Read the model definition and answer for the solid it produces. Units are mm, in the model's axes. Face numbers are marked on the shaded views. A direction names the side the tool comes from. Coordinates: 2 decimals unless noted, no trailing zeros. Loops run counter-clockwise (first coordinate to the right, second up) from the corner with the lowest first, then second, coordinate; pieces in that order, holes last. Notation, with made-up numbers: (30, -3.75) -> (54, -3.75) arc R21 ccw to (54, 34.25) -> close; hole circle Ø7 at (25.25, 83.25). An arc over 180 degrees is marked (long way). Answer in a Markdown table with one row per item.
```python
from build123d import *

# Parameters (mm, degrees)
ESQUISSE1_R          = 2
ESQUISSE1_R_2        = 1.5
BOSS_EXTRU_1_DEPTH   = 39.58852
BOSS_EXTRU_1_2_DEPTH = 39.58852
BOSS_EXTRU_2_DEPTH   = 20


with BuildPart() as part:
    # Esquisse1 → Boss.-Extru.1 (new body)
    with BuildSketch(Plane.XY):
        with Locations(Location((0, 3.882050808, 0), (0, 0, 180))):
            Circle(ESQUISSE1_R)
        with Locations(Location((0, 3.882050808, 0), (0, 0, 180))):
            Circle(ESQUISSE1_R_2, mode=Mode.SUBTRACT)
    extrude(amount=BOSS_EXTRU_1_DEPTH)



with BuildPart() as body_2:
    # Esquisse1 → Boss.-Extru.1 2 (new body)
    with BuildSketch(Plane.XY):
        with Locations(Location((0, -3.882050808, 0), (0, 0, 180))):
            Circle(ESQUISSE1_R)
        with Locations((0, -3.882050808)):
            Circle(ESQUISSE1_R_2, mode=Mode.SUBTRACT)
    extrude(amount=BOSS_EXTRU_1_2_DEPTH)


with BuildPart() as part_1:
    add(part.part)

    add(body_2.part)  # Boss.-Extru.2 merges body 2
    # Esquisse1<3> → Boss.-Extru.2 (add)
    with BuildSketch(Plane.XY):
        with BuildLine():
            ThreePointArc((-1, -2.15), (0, -1.882050808), (1, -2.15))
            Line((1, -2.15), (1, 2.15))
            ThreePointArc((1, 2.15), (0, 1.882050808), (-1, 2.15))
            Line((-1, 2.15), (-1, -2.15))
        make_face()
    extrude(amount=BOSS_EXTRU_2_DEPTH)


solid = part_1.part
```
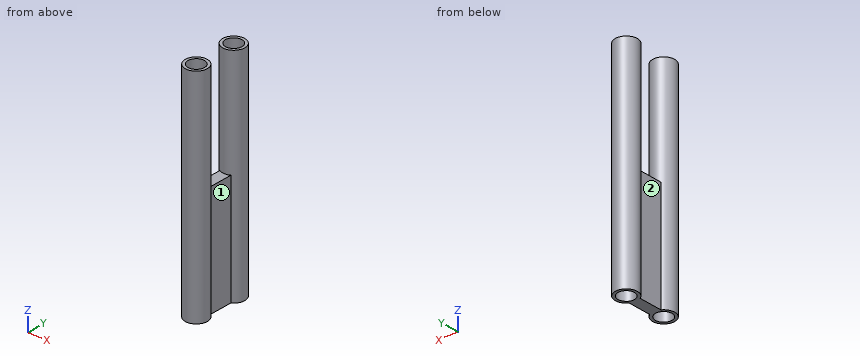
1. A cutting plane is placed at D-D on z = 37. Give the vertices of the cut face in (x, y), and give its area (3 significant figures).
A:
| item | result |
|---|---|
| outline | circle Ø4 at (0, -3.88); circle Ø4 at (0, 3.88); hole circle Ø3 at (0, -3.88); hole circle Ø3 at (0, 3.88) |
| area | 11.0 mm2 |
2. A cutting plane is placed at B-B on y = -3.5. Give the vertices of the cut face in (x, z).
A:
| item | result |
|---|---|
| outline | (-1.96, 0) -> (-1.45, 0) -> (-1.45, 39.59) -> (-1.96, 39.59) -> close; (1.45, 0) -> (1.96, 0) -> (1.96, 39.59) -> (1.45, 39.59) -> close |
3. A cutting plane is placed at A-A on x = 0. Give the vertices of the cut face in (y, z), and give its area (3 significant figures).
A:
| item | result |
|---|---|
| outline | (-5.88, 0) -> (-5.38, 0) -> (-5.38, 39.59) -> (-5.88, 39.59) -> close; (-2.38, 0) -> (2.38, 0) -> (2.38, 39.59) -> (1.88, 39.59) -> (1.88, 20) -> (-1.88, 20) -> (-1.88, 39.59) -> (-2.38, 39.59) -> close; (5.38, 0) -> (5.88, 0) -> (5.88, 39.59) -> (5.38, 39.59) -> close |
| area | 154 mm2 |
4. Given pin 1 Ø1.3 at (y, z) = (-0.5, 13) entering from -X; pin 2 Ø2 at (y, z) = (-3, 16.5) entering from -X; pin 3 Ø2 at (y, z) = (-0.5, 12.5) entering from +X, each flat-ended and moving along its own axis, determine where each tip first touches the part or whether it passes through.
A:
| item | result |
|---|---|
| pin 1 | stops at x = -1 |
| pin 2 | stops at x = -2 |
| pin 3 | stops at x = 1 |
5. A cutting plane is placed at C-C on z = 13. Give the vertices of the cut face in (x, y), and give its area (3 significant figures).
A:
| item | result |
|---|---|
| outline | (-1, -2.15) arc R2 ccw (long way) to (1, -2.15) -> (1, 2.15) arc R2 ccw (long way) to (-1, 2.15) -> close; hole circle Ø3 at (0, -3.88); hole circle Ø3 at (0, 3.88) |
| area | 18.9 mm2 |
6. A tool of negligible diameter and unlimited length cuts with its end or side. For the marked faces 1 and 2, from which of +Z, -Z, +X, -X, +Y, -Y can it reach the whole face along a straight path? Write none if from no direction.
A:
| item | result |
|---|---|
| face 1 | +Z, -Z, +X |
| face 2 | +Z, -Z, -X |
7. Find the intervals of material crossed by probe 1 along Y at (x, z) = (0, 25); probe 2 along Y at (x, z) = (0.65, 30.5); probe 3 along Y at (x, z) = (0, 9), in increasing order.
A:
| item | result |
|---|---|
| probe 1 | y = -5.88 to -5.38, -2.38 to -1.88, 1.88 to 2.38, 5.38 to 5.88 |
| probe 2 | y = -5.77 to -5.23, -2.53 to -1.99, 1.99 to 2.53, 5.23 to 5.77 |
| probe 3 | y = -5.88 to -5.38, -2.38 to 2.38, 5.38 to 5.88 |
